Check sheet for the modelled part. Datum: model origin and axes. Units: mm. Face numbers are marked on the shaded views. A direction names the side the tool comes from. Round coordinates to 2 decimals unless told otherwise and drop trailing zeros. Loops run counter-clockwise (first coordinate to the right, second up) from the corner with the lowest first, then second, coordinate; pieces in that order, holes last. Notation, with made-up numbers: (-26, 11.25) -> (-12, 11.25) arc R11 ccw to (-12, 21.25) -> close; hole circle Ø1 at (-3, 42). An arc over 180 degrees is marked (long way). Use one line per item in the form item = value. Start each with the question number.
(1) Sectioned sample at A-A (x = 66). Record the cut outline in (y, z), and give its area (3 significant figures).
(2) Sectioned sample at C-C (x = -32). Record the cut outline in (y, z), and give its area (3 significant figures).
(3) Set-up check for the marked faces 1 and 2: record each of +Z, -Z, +X, -X, +Y, -Y from which the full face is reachable in a straight line by a thin tool's end or side.
(4) Draft check along X on the marked faces 3, 4 and 5. Enter one of: released by +X, released by -X, zero draft, split by the parting line, or undercut.
(5) Go/stop test with flat-tipped pins: pin 1 (3.5 mm diameter, centred on y = 29.5, z = 22.5, fed in from -X); pin 2 (1.6 mm diameter, centred on x = -14.5, z = 5.5, fed in from -Y). Record where each tip stops, or that it passes through.
(6) Sectioned sample at B-B (y = 29.5). Record the cut outline in (x, z) (3 decimals), and give its area (3 significant figures).
(7) Material ranges on probe 1 along Z at (x, y) = (13.5, 29.95); probe 2 along X at (y, z) = (28.75, 4); probe 3 along X at (y, z) = (30.5, 4.5), recorded low to high. Write a range as [from, to].
Autodesk Inventor part; units mm, degrees
ref_plane "YZ Plane" through (0, 0, 0) normal (1, 0, 0) x (0, 1, 0)
ref_plane "XZ Plane" through (0, 0, 0) normal (0, 1, 0) x (-1, 0, 0)
ref_plane "XY Plane" through (0, 0, 0) normal (0, 0, 1) x (1, 0, 0)
sketch "Sketch1" plane through (0, 0, 0) normal (0, 0, 1) x (1, 0, 0)
  line L0 (91, -34) -> (91, 34)
  line L1 (91, 34) -> (41, 34)
  line L2 (41, 34) -> (41, 89)
  line L3 (41, 89) -> (-91, 89)
  line L4 (-91, 89) -> (-91, -89)
  line L5 (-91, -89) -> (41, -89)
  line L6 (41, -89) -> (41, -34)
  line L7 (41, -34) -> (91, -34)
  line L8 (70, 27) -> (62, 27)
  line L9 (91, 34) -> (-87, 34)
  line L10 (-87, 34) -> (-87, 27)
  line L11 (-87, 27) -> (91, 27)
  line L12 (91, 27) -> (91, 34)
  circle A0 centre (-83, 21.5) radius 1.2295
  circle A1 centre (-83, -64.5) radius 1.2295
  circle A2 centre (-83, -21.5) radius 1.2295
  circle A3 centre (-83, 64.5) radius 1.2295
  line L13 (-85, -72) -> (-76, -72)
  line L14 (-76, -72) -> (-76, -57)
  line L15 (-76, -57) -> (-85, -57)
  arc A4 (-87, -55) -> (-85, -57) centre (-85, -55) ccw
  line L16 (-87, -55) -> (-87, -31)
  arc A5 (-85, -29) -> (-87, -31) centre (-85, -31) ccw
  line L17 (-85, -29) -> (-76, -29)
  line L18 (-76, -29) -> (-76, -14)
  line L19 (-76, -14) -> (-85, -14)
  arc A6 (-87, -12) -> (-85, -14) centre (-85, -12) ccw
  line L20 (-87, -12) -> (-87, 12)
  arc A7 (-85, 14) -> (-87, 12) centre (-85, 12) ccw
  line L21 (-85, 14) -> (-76, 14)
  line L22 (-76, 14) -> (-76, 29)
  line L23 (-76, 29) -> (-85, 29)
  arc A8 (-87, 31) -> (-85, 29) centre (-85, 31) ccw
  line L24 (-87, 31) -> (-87, 55)
  arc A9 (-85, 57) -> (-87, 55) centre (-85, 55) ccw
  line L25 (-85, 57) -> (-76, 57)
  line L26 (-76, 57) -> (-76, 72)
  line L27 (-76, 72) -> (-85, 72)
  arc A10 (-87, 74) -> (-85, 72) centre (-85, 74) ccw
  line L28 (-87, 74) -> (-87, 89)
  line L29 (-91, 89) -> (-87, 89)
  line L30 (-91, -89) -> (-91, 89)
  line L31 (-91, -89) -> (-87, -89)
  line L32 (-87, -89) -> (-87, -74)
  arc A11 (-85, -72) -> (-87, -74) centre (-85, -74) ccw
  line L33 (-91, 89.5) -> (-86.5, 89.5)
  line L34 (-86.5, 89.5) -> (-86.5, 74)
  arc A12 (-86.5, 74) -> (-85, 72.5) centre (-85, 74) ccw
  line L35 (-85, 72.5) -> (-75.5, 72.5)
  line L36 (-75.5, 72.5) -> (-75.5, 56.5)
  line L37 (-75.5, 56.5) -> (-85, 56.5)
  arc A13 (-85, 56.5) -> (-86.5, 55) centre (-85, 55) ccw
  line L38 (-86.5, 55) -> (-86.5, 31)
  arc A14 (-86.5, 31) -> (-85, 29.5) centre (-85, 31) ccw
  line L39 (-85, 29.5) -> (-75.5, 29.5)
  line L40 (-75.5, 29.5) -> (-75.5, 13.5)
  line L41 (-75.5, 13.5) -> (-85, 13.5)
  arc A15 (-85, 13.5) -> (-86.5, 12) centre (-85, 12) ccw
  line L42 (-86.5, 12) -> (-86.5, -12)
  arc A16 (-86.5, -12) -> (-85, -13.5) centre (-85, -12) ccw
  line L43 (-85, -13.5) -> (-75.5, -13.5)
  line L44 (-75.5, -13.5) -> (-75.5, -29.5)
  line L45 (-75.5, -29.5) -> (-85, -29.5)
  arc A17 (-85, -29.5) -> (-86.5, -31) centre (-85, -31) ccw
  line L46 (-86.5, -31) -> (-86.5, -55)
  arc A18 (-86.5, -55) -> (-85, -56.5) centre (-85, -55) ccw
  line L47 (-85, -56.5) -> (-75.5, -56.5)
  line L48 (-75.5, -56.5) -> (-75.5, -72.5)
  line L49 (-75.5, -72.5) -> (-85, -72.5)
  arc A19 (-85, -72.5) -> (-86.5, -74) centre (-85, -74) ccw
  line L50 (-86.5, -74) -> (-86.5, -89.5)
  line L51 (-86.5, -89.5) -> (-91, -89.5)
  line L52 (-86.5, 31) -> (-75.5, 31)
  line L53 (-75.5, 31) -> (-75.5, 29.5)
  line L54 (-75.5, 31) -> (-75.5, 34)
  point P0 (0, 0)
  point P1 (-75.5, 27)
  point P2 (-86.5, 34)
  dimension "d6" = 0.5
extrude "Extrusion1" add sketch "Sketch1" along normal blind 30 contours L11 L8 L40 L53 L54 L9 L1 L0
sketch "Sketch3" plane through (-86.5, 34, 0) normal (0, 1, 0) x (1, 0, 0)
  line L0 (-0.5, -4.5) -> (-0.5, 0)
  line L1 (-0.5, 0) -> (-4.5, 0)
  line L2 (-4.5, 0) -> (-4.5, 3.5)
  line L3 (-4.5, 3.5) -> (-18.5, 3.5)
  line L4 (-18.5, 3.5) -> (-4.5, -5.5)
  line L5 (-4.5, -5.5) -> (-4.5, -4.5)
  line L6 (-4.5, -4.5) -> (-0.5, -4.5)
  line L7 (-0.5, -4.5) -> (50.0525, -33.6865)
  line L8 (177.5, 0) -> (11, 0)
  line L9 (177.5, -30) -> (11, -30)
  line L10 (177.5, 0) -> (177.5, -30)
  line L11 (11, 0) -> (11, -30)
  point P0 (86.5, 0)
  point P1 (43.6673, -30)
  point P2 (11, -11.1395)
  dimension "d7" = 30
extrude "Extrusion4" cut sketch "Sketch3" against normal blind 30 contours L7 L9 L11
sketch "Sketch5" plane through (-75.5, 27, 0) normal (0, -1, 0) x (1, 0, 0)
  line L0 (56.5, 7.0341) -> (57.5, 7.0341)
  line L1 (34.5, 7.0341) -> (56.5, 7.0341)
  line L2 (33.5, 7.0341) -> (33.5, 6.6226)
  line L3 (33.5, 6.6226) -> (9.5, 6.6226)
  line L4 (9.5, 6.6226) -> (9.5, 7.0341)
  line L5 (9.5, 7.0341) -> (33.5, 7.0341)
  line L6 (64.5, 7.0341) -> (64.5, 6.6226)
  line L7 (64.5, 6.6226) -> (57.5, 6.6226)
  line L8 (57.5, 6.6226) -> (57.5, 7.0341)
  line L9 (57.5, 7.0341) -> (64.5, 7.0341)
  line L10 (9.5, 2) -> (9.5, 2.6226)
  line L11 (9.5, 2.6226) -> (64.5, 2.6226)
  line L12 (64.5, 2.6226) -> (64.5, 2)
  line L13 (64.5, 2) -> (9.5, 2)
  line L14 (9.5, 7.0341) -> (64.5, 7.0341)
  line L15 (64.5, 7.0341) -> (64.5, 2)
  line L16 (64.5, 2) -> (9.5, 2)
  line L17 (9.5, 2) -> (9.5, 7.0341)
  line L18 (9.2, 7.3341) -> (64.8, 7.3341)
  line L19 (64.8, 7.3341) -> (64.8, 1.9)
  line L20 (64.8, 1.9) -> (9.2, 1.9)
  line L21 (9.2, 1.9) -> (9.2, 7.3341)
  point P0 (75.5, 0)
  dimension "d19" = 0.3
  dimension "d20" = 0.3
  dimension "d21" = 0.1
  dimension "d22" = 0.3
extrude "Extrusion6" cut sketch "Sketch5" against normal blind 0.7 contours L0 L8 L7 L15 L11 L17 L3 L2 L14 L1 | L9 L6 L7 L8 | L2 L3 L4 L5 | L12 L13 L10 L11 | L18 L19 L20 L21
sketch "Sketch6" plane through (-75.5, 27, 0) normal (0, -1, 0) x (1, 0, 0)
  line L0 (33.5, 7.0341) -> (34.5, 7.0341)
  line L1 (34.5, 7.0341) -> (56.5, 7.0341)
  line L2 (56.5, 7.0341) -> (57.5, 7.0341)
  line L3 (64.8, 1.9) -> (9.2, 1.9)
  line L4 (64.8, 7.3341) -> (64.8, 1.9)
  line L5 (9.2, 7.3341) -> (64.8, 7.3341)
  line L6 (9.2, 1.9) -> (9.2, 7.3341)
  line L7 (33.5, 7.3341) -> (57.5, 7.3341)
  line L8 (57.5, 7.3341) -> (57.5, 1.9)
  line L9 (57.5, 1.9) -> (33.5, 1.9)
  line L10 (33.5, 1.9) -> (33.5, 7.3341)
  point P0 (75.5, 0)
extrude "Extrusion7" cut sketch "Sketch6" against normal up to next contours L10 L5 L8 L2 L1 L0 | L0 L1 L2 L8 L3 L10
sketch "Sketch7" plane through (0, 0, 30) normal (0, 0, 1) x (1, 0, 0)
  line L0 (10.25, -34) -> (10.25, 34)
  line L1 (10.25, 34) -> (-5.75, 34)
  line L2 (-5.75, -34) -> (-5.75, 34)
  line L3 (10.25, -34) -> (-5.75, -34)
  line L4 (-42.8327, 27) -> (91, 27)
  line L5 (10.25, 34) -> (-5.75, 34)
  line L6 (-5.75, 34) -> (-5.75, 27)
  line L7 (-5.75, 27) -> (10.25, 27)
  line L8 (10.25, 27) -> (10.25, 34)
  line L9 (10.65, 34) -> (-6.15, 34)
  line L10 (-6.15, 34) -> (-6.15, 27)
  line L11 (-6.15, 27) -> (10.65, 27)
  line L12 (10.65, 27) -> (10.65, 34)
  point P0 (0, 0)
  dimension "d27" = 0.4
  dimension "d28" = 0.4
extrude "Extrusion8" cut sketch "Sketch7" against normal blind 15.5 contours L4 L2 L1 L0 | L0 L9 L12 L4 | L4 L10 L9 L2
sketch "Sketch8" plane through (-75.5, 27, 0) normal (0, -1, 0) x (1, 0, 0)
  circle A0 centre (89, 3.25) radius 1.8
  circle A1 centre (113.25, 3.25) radius 1.8
  point P0 (75.5, 0)
hole "Hole1" at (13.5, 27, 3.25) at (37.75, 27, 3.25) direction (0, 1, 0) diameter 3.6 end through all countersink diameter 6.5 countersink angle 90
sketch "Sketch9" plane through (91, 27, 0) normal (0, -1, 0) x (1, 0, 0)
  arc A0 (-67.8175, 18.3693) -> (-69.7313, 19.2694) centre (-70.7618, 14.5935) ccw
  arc A1 (-69.7313, 19.2694) -> (-70.2869, 18.54) centre (-65.375, 15.375) ccw
  arc A2 (-70.2869, 18.54) -> (-68.9106, 16.9341) centre (-66.053, 20.7758) ccw
  arc A3 (-68.9106, 16.9341) -> (-69.111, 16.3618) centre (-65.375, 15.375) ccw
  arc A4 (-69.111, 16.3618) -> (-71.1884, 15.965) centre (-69.2737, 11.5765) ccw
  arc A5 (-71.1884, 15.965) -> (-71.2091, 15.0484) centre (-65.375, 15.375) ccw
  arc A6 (-71.2091, 15.0484) -> (-69.1518, 14.5581) centre (-69.098, 19.3459) ccw
  arc A7 (-69.1518, 14.5581) -> (-68.9775, 13.9774) centre (-65.375, 15.375) ccw
  arc A8 (-68.9775, 13.9774) -> (-70.425, 12.4353) centre (-66.2964, 10.0103) ccw
  arc A9 (-70.425, 12.4353) -> (-69.9029, 11.6815) centre (-65.375, 15.375) ccw
  arc A10 (-69.9029, 11.6815) -> (-67.9503, 12.4942) centre (-70.721, 16.3992) ccw
  arc A11 (-67.9503, 12.4942) -> (-67.468, 12.1268) centre (-65.375, 15.375) ccw
  arc A12 (-67.468, 12.1268) -> (-67.7326, 10.0285) centre (-62.9672, 10.4933) ccw
  arc A13 (-67.7326, 10.0285) -> (-66.8672, 9.7255) centre (-65.375, 15.375) ccw
  arc A14 (-66.8672, 9.7255) -> (-65.7652, 11.5306) centre (-70.302, 13.0613) ccw
  arc A15 (-65.7652, 11.5306) -> (-65.159, 11.5169) centre (-65.375, 15.375) ccw
  arc A16 (-65.159, 11.5169) -> (-64.1397, 9.6638) centre (-60.5576, 12.8409) ccw
  arc A17 (-64.1397, 9.6638) -> (-63.2615, 9.9273) centre (-65.375, 15.375) ccw
  arc A18 (-63.2615, 9.9273) -> (-63.431, 12.0355) centre (-68.0011, 10.6071) ccw
  arc A19 (-63.431, 12.0355) -> (-62.9325, 12.3807) centre (-65.375, 15.375) ccw
  arc A20 (-62.9325, 12.3807) -> (-61.0187, 11.4806) centre (-59.9882, 16.1565) ccw
  arc A21 (-61.0187, 11.4806) -> (-60.4631, 12.21) centre (-65.375, 15.375) ccw
  arc A22 (-60.4631, 12.21) -> (-61.8394, 13.8159) centre (-64.697, 9.9742) ccw
  arc A23 (-61.8394, 13.8159) -> (-61.639, 14.3882) centre (-65.375, 15.375) ccw
  arc A24 (-61.639, 14.3882) -> (-59.5616, 14.785) centre (-61.4763, 19.1735) ccw
  arc A25 (-59.5616, 14.785) -> (-59.5409, 15.7016) centre (-65.375, 15.375) ccw
  arc A26 (-59.5409, 15.7016) -> (-61.5982, 16.1919) centre (-61.652, 11.4041) ccw
  arc A27 (-61.5982, 16.1919) -> (-61.7725, 16.7726) centre (-65.375, 15.375) ccw
  arc A28 (-61.7725, 16.7726) -> (-60.325, 18.3147) centre (-64.4536, 20.7397) ccw
  arc A29 (-60.325, 18.3147) -> (-60.8471, 19.0685) centre (-65.375, 15.375) ccw
  arc A30 (-60.8471, 19.0685) -> (-62.7997, 18.2558) centre (-60.029, 14.3508) ccw
  arc A31 (-62.7997, 18.2558) -> (-63.282, 18.6232) centre (-65.375, 15.375) ccw
  arc A32 (-63.282, 18.6232) -> (-63.0174, 20.7215) centre (-67.7828, 20.2567) ccw
  arc A33 (-63.0174, 20.7215) -> (-63.8828, 21.0245) centre (-65.375, 15.375) ccw
  arc A34 (-63.8828, 21.0245) -> (-64.9848, 19.2194) centre (-60.448, 17.6887) ccw
  arc A35 (-64.9848, 19.2194) -> (-65.591, 19.2331) centre (-65.375, 15.375) ccw
  arc A36 (-65.591, 19.2331) -> (-66.6103, 21.0862) centre (-70.1924, 17.9091) ccw
  arc A37 (-66.6103, 21.0862) -> (-67.4885, 20.8227) centre (-65.375, 15.375) ccw
  arc A38 (-67.4885, 20.8227) -> (-67.319, 18.7145) centre (-62.7489, 20.1429) ccw
  arc A39 (-67.319, 18.7145) -> (-67.8175, 18.3693) centre (-65.375, 15.375) ccw
  circle A40 centre (-65.375, 15.375) radius 5.8433
  circle A41 centre (-65.375, 15.375) radius 6.8433
  circle A42 centre (-25, 8.5) radius 5.5
  point P0 (-91, 0)
  dimension "d38" = 1
extrude "Extrusion9" cut sketch "Sketch9" against normal up to next contours A39 A38 A37 A36 A35 A34 A33 A32 A31 A30 A29 A28 A27 A26 A25 A24 A23 A22 A21 A20 A19 A18 A17 A16 A15 A14 A13 A12 A11 A10 A9 A8 A7 A6 A5 A4 A3 A2 A1 A0 | A0 A40 A38 A39 | A2 A3 A4 A40 | A40 A34 A35 A36 | A6 A7 A8 A40 | A40 A30 A31 A32 | A10 A11 A12 A40 | A40 A26 A27 A28 | A14 A15 A16 A40 | A18 A19 A20 A40 | A40 A22 A23 A24 | A41
sketch "Sketch10" plane through (91, 27, 0) normal (0, -1, 0) x (1, 0, 0)
  circle A0 centre (-25, 8.5) radius 5.5
  circle A1 centre (-25, 8.5) radius 5.7
  point P0 (-91, 0)
  dimension "d41" = 0.2
extrude "Extrusion10" cut sketch "Sketch10" against normal blind 6 contours A0 | A1
sketch "Sketch11" plane through (-75.5, 34, 0) normal (0, 1, 0) x (1, 0, 0)
  circle A0 centre (141.5, -8.5) radius 1.2295
  line L0 (143.8461, -6.6303) -> (139.813, -6.0193)
  arc A1 (139.813, -6.0193) -> (139.1539, -10.3697) centre (141.5, -8.5) ccw
  line L1 (139.1539, -10.3697) -> (143.187, -10.9807)
  arc A2 (143.187, -10.9807) -> (143.8461, -6.6303) centre (141.5, -8.5) ccw
  circle A3 centre (141.5, -8.5) radius 5.7
  circle A4 centre (141.5, -8.5) radius 3
  circle A5 centre (141.5, -8.5) radius 3.4
  point P0 (75.5, 0)
  dimension "d44" = 0.4
extrude "Extrusion11" cut sketch "Sketch11" against normal blind 6 contours A0 | A2 L1 A1 L0 | L0 A4 | L1 A4 | A5
properties part number "right_hold"
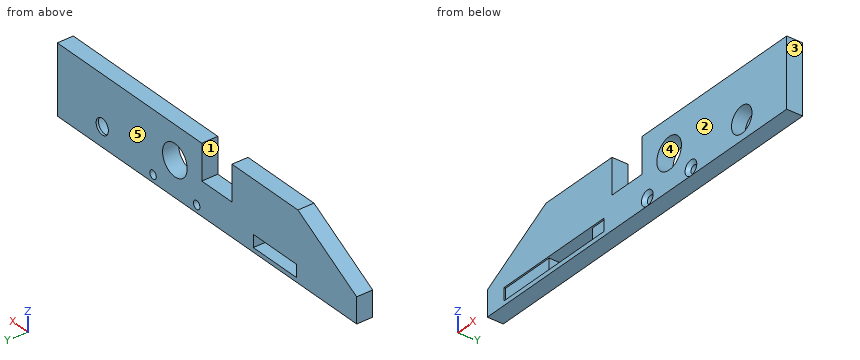
Checks:
q1.outline = (27, 0) -> (34, 0) -> (34, 5.1) -> (33, 5.1) -> (33, 2.8) -> (27, 2.8) -> close; (27, 14.2) -> (33, 14.2) -> (33, 11.9) -> (34, 11.9) -> (34, 30) -> (27, 30) -> close
q1.area = 135 mm2
q2.outline = (27, 0) -> (34, 0) -> (34, 1.9) -> (27, 1.9) -> close; (27, 7.33) -> (34, 7.33) -> (34, 30) -> (27, 30) -> close
q2.area = 172 mm2
q3.face_1 = +Z, +Y, -Y
q3.face_2 = +Z, -Z, +X, -X, -Y
q4.face_3 = released by +X
q4.face_4 = undercut
q4.face_5 = zero draft
q5.pin_1 = -58.85
q5.pin_2 = 27.7
q6.outline = (-75.5, 0) -> (91, 0) -> (91, 30) -> (10.65, 30) -> (10.65, 14.5) -> (-6.15, 14.5) -> (-6.15, 30) -> (-42.833, 30) -> (-75.5, 11.14) -> close; hole (-42, 1.9) -> (-18, 1.9) -> (-18, 7.334) -> (-42, 7.334) -> close; hole circle Ø3.6 at (13.5, 3.25); hole circle Ø13.687 at (25.625, 15.375); hole circle Ø3.6 at (37.75, 3.25); hole circle Ø11.4 at (66, 8.5)
q6.area = 4,030 mm2
q7.probe_1 = [0, 1.45], [5.05, 30]
q7.probe_2 = [-75.5, -42], [-18, 11.86], [15.14, 36.11], [39.39, 62.5], [69.5, 91]
q7.probe_3 = [-75.5, -42], [-18, 12.2], [14.8, 36.45], [39.05, 61.94], [70.06, 91]
